Autodesk Inventor part; units mm, degrees
ref_plane "YZ Plane" through (0, 0, 0) normal (1, 0, 0) x (0, 1, 0)
ref_plane "XZ Plane" through (0, 0, 0) normal (0, 1, 0) x (-1, 0, 0)
ref_plane "XY Plane" through (0, 0, 0) normal (0, 0, 1) x (1, 0, 0)
sketch "Sketch1" plane through (0, 0, 0) normal (0, 0, 1) x (1, 0, 0)
  line L0 (-12.7, -12.7) -> (12.7, -12.7)
  line L1 (12.7, -12.7) -> (12.7, 12.7)
  line L2 (12.7, 12.7) -> (-12.7, 12.7)
  line L3 (-12.7, 12.7) -> (-12.7, -12.7)
  line L4 (-9.525, 9.525) -> (9.525, 9.525)
  line L5 (9.525, 9.525) -> (9.525, -9.525)
  line L6 (9.525, -9.525) -> (-9.525, -9.525)
  line L7 (-9.525, -9.525) -> (-9.525, 9.525)
  arc A0 (-9.525, 9.525) -> (-12.7, 12.7) centre (-12.7, 9.525) ccw
  arc A1 (12.7, -12.7) -> (9.525, -9.525) centre (9.525, -12.7) ccw
  point P0 (0, 0)
  point P1 (-12.7, 0)
  point P2 (0, 12.7)
  dimension "d0" = 25.4
  dimension "d1" = 25.4
  dimension "d2" = 3.175
extrude "Extrusion1" add sketch "Sketch1" along normal mid plane 342.9 contours L3 A0 L7 L6 A1 L0
sketch "Sketch2" plane through (-9.525, -9.525, 171.45) normal (1, 0, 0) x (0, 0, -1)
  line L0 (342.9, -3.175) -> (0, -3.175)
  line L1 (0, 22.225) -> (0, -3.175)
  line L2 (342.9, 22.225) -> (0, 22.225)
  line L3 (342.9, -3.175) -> (342.9, 22.225)
  line L4 (0, 9.525) -> (342.9, 9.525)
  point P0 (171.45, 9.525)
  point P1 (25.4, 9.525)
  point P2 (76.2, 9.525)
  point P3 (171.45, 9.525)
  point P4 (266.7, 9.525)
  point P5 (317.5, 9.525)
  dimension "d5" = 12.7
  dimension "d6" = 25.4
  dimension "d7" = 50.8
  dimension "d8" = 25.4
  dimension "d9" = 50.8
hole "Hole1" at (-9.525, 0, 146.05) at (-9.525, 0, 95.25) at (-9.525, 0, 0) at (-9.525, 0, -95.25) at (-9.525, 0, -146.05) direction (-1, 0, 0) diameter 4.5 depth 12.446 tip angle 118
properties part number "1213_Angle Stock Bracket_V1" material "Aluminum"
Read the model definition and answer for the solid it produces. Units are mm, in the model's axes. A direction names the side the tool comes from. Give positions to 0.01 mm unless a question says otherwise; leave off trailing zeros. Write each loop counter-clockwise with the first axis right and the second up, starting at its lowest first coordinate (ties: lowest second). Pieces come first, ordered by that corner, then holes. Notation, with made-up numbers: (64.25, -9) - (108.25, -9) arc R23 cw to (108.25, 13) - close; hole circle Ø10 at (17, 21). An arc over 180 degrees is marked (long way). Answer in a Markdown table with one row per item. Add a question column.
Item 1: Section A-A, the plane z = 129 is taken. Write down the section's boundary in (x, y) (3 decimals).
Item 2: Find the intervals of material crossed by L1, parallel to Z at x = -10.9, y = 0; L2, parallel to Y at x = 7.75, z = 28.5 (3 decimals), in increasing order.
Item 3: Flat-ended cylindrical pins translate along their axes: P1, Ø7, axis at y = 0, z = -95.25, coming from the +X side (3 decimals); P2, Ø5.5, axis at x = -1, z = 35.5, coming from the +Y side (3 decimals). Find the tip coordinate at first contact, or state that the pin passes through.
Item 4: A tool of negligible diameter and unlimited length cuts with its end or side. For faces 4 (the face through (-9.525, -0.1, -2.4)), 5 (the face through (-10, -5, 171.45)), from which of +Z, -Z, +X, -X, +Y, -Y can it reach the whole face along a straight path? Write none if from no direction.
Item 5: Section B-B, the plane x = -3 is taken. Write down the section's boundary in (y, z) (3 decimals).
Item 6: Determine the mould class of faces 1 (the face through (0, -9.525, -2)), 2 (the face through (-12.7, 0.2, -2.4)), 3 (the face through (0, -12.7, -2)) for opening direction Y: pulls with the +Y half, pulls with the -Y half, needs draft (parallel to the pull), parting line crosses it, or undercut.
Recorded:
| question | item | result |
|---|---|---|
| 1 | outline | (-12.7, -12.7) - (12.7, -12.7) arc R3.175 ccw to (9.525, -9.525) - (-9.525, -9.525) - (-9.525, 9.525) arc R3.175 ccw to (-12.7, 12.7) - close |
| 2 | L1 | z = -171.45 to -148.3, -143.8 to -97.5, -93 to -2.25, 2.25 to 93, 97.5 to 143.8, 148.3 to 171.45 |
| 2 | L2 | y = -12.7 to -9.525 |
| 3 | P1 | stops at x = -9.525 |
| 3 | P2 | stops at y = -9.525 |
| 4 | face 4 | +Z, -Z, +X, +Y |
| 4 | face 5 | +Z, +X, -X, +Y, -Y |
| 5 | outline | (-12.7, -171.45) - (-9.525, -171.45) - (-9.525, 171.45) - (-12.7, 171.45) - close |
| 6 | face 1 | pulls with the +Y half |
| 6 | face 2 | needs draft |
| 6 | face 3 | pulls with the -Y half |
